from build123d import *

# Parameters (mm, degrees)
SKETCH1_R                     = 9.398
BOSS_EXTRUDE1_DEPTH           = 12.7
TAP_DRILL_FOR_8_32_TAP1_D     = 3.4544
TAP_DRILL_FOR_8_32_TAP1_DEPTH = 10.16
TAP_DRILL_FOR_8_32_TAP1_TIP   = 1.037806461


with BuildPart() as part:
    # Sketch1 → Boss-Extrude1 (new body)
    with BuildSketch(Plane(origin=(0, 0, 0), x_dir=(1, 0, 0), z_dir=(0, 1, 0))):
        Circle(SKETCH1_R)
    extrude(amount=BOSS_EXTRUDE1_DEPTH)

    # Sketch3 → Revolve1 (revolve)
    with BuildSketch(Plane(origin=(0, 0, 0), x_dir=(0, 0, -1), z_dir=(1, 0, 0))):
        with BuildLine():
            Line((0, 12.7), (12.065, 12.7))
            Line((12.065, 12.7), (1.27, 167.075692241))
            Line((1.27, 167.075692241), (1.257640447, 167.252442079))
            ThreePointArc((1.257640447, 167.252442079), (0.833194967, 168.034173408), (0, 168.345692241))
            Line((0, 168.345692241), (0, 12.7))
        make_face()
    revolve(axis=Axis((0, 185.237538387, 0), (0, -1, 0)))

    # Tap Drill for #8-32 Tap1
    with Locations(Plane(origin=(0, 0, 0), x_dir=(-1, 0, 0), z_dir=(0, -1, 0))):
        with Locations((0, 0)):
            Hole(TAP_DRILL_FOR_8_32_TAP1_D / 2, depth=TAP_DRILL_FOR_8_32_TAP1_DEPTH)
            with Locations((0, 0, -(TAP_DRILL_FOR_8_32_TAP1_DEPTH + TAP_DRILL_FOR_8_32_TAP1_TIP / 2))):  # 118° drill point
                Cone(0, TAP_DRILL_FOR_8_32_TAP1_D / 2, TAP_DRILL_FOR_8_32_TAP1_TIP, mode=Mode.SUBTRACT)


solid = part.part
Can you work these out from the model? Positions are in its coordinate system, mm. Coordinates: 2 decimals unless noted, no trailing zeros. Loops run counter-clockwise (first coordinate to the right, second up) from the corner with the lowest first, then second, coordinate; pieces in that order, holes last. Notation, with made-up numbers: M 67,-28 L 75,-28 A29 cw 75,2 Z; hole C 85,67 d8. An arc over 180 degrees is marked long. Return JSON: item names as keys, results as strings. Group by question number.
Item 1: Imagine slicing it at B-B (y = 85). Please give me the cut outline in (x, z), and give its area (3 significant figures).
Item 2: Imagine slicing it at A-A (y = 111.5). Please give me the cut outline in (x, z), and give its area (3 significant figures).
Item 3: If I drill on L1, parallel to Z at x = 0, y = 4; L2, parallel to X at y = 58.5, z = 1.75; L3, parallel to X at y = 90, z = 5, over which ranges is the centre line in solid material (lowest first)? Write a range as from..to.
Item 4: I'm going to push flat-ended pins straight in: pin 1 Ø12 at (y, z) = (96.5, -6) entering from -X; pin 2 Ø1.5 at (x, y) = (2.5, 24) entering from -Z; pin 3 Ø2 at (y, z) = (146, -5) entering from -X; pin 4 Ø5 at (x, y) = (3.5, 29) entering from -Z. Where does each tip first touch, or does it pass through?
Item 5: Thinking about a two-plate mould opening in X: for faces 1 (the cylindrical face through (-1.22, 6.26, -9.32)), 2 (the cylindrical face through (-0.225, 5.151, -1.713)), 3 (the flat face through (2, 0, 0)), which applies, released by +X, released by -X, zero draft, split by the parting line, or undercut?
Verdict:
{
 "1": {"outline": "C 0,0 d14.02", "area": "154 mm^2"},
 "2": {"outline": "C 0,0 d10.31", "area": "83.5 mm^2"},
 "3": {"L1": "z = -9.4..-1.73, 1.73..9.4", "L2": "x = -8.69..8.69", "L3": "x = -4.4..4.4"},
 "4": {"pin 1": "stops at x = -6.36", "pin 2": "stops at z = -11.15", "pin 3": "passes through", "pin 4": "stops at z = -10.93"},
 "5": {"face 1": "split by the parting line", "face 2": "undercut", "face 3": "zero draft"}
}
